Part print with two shaded views. Sizes in mm from the minimum x, y, z corner. Give positions to 0.01 mm unless a question says otherwise; leave off trailing zeros. Loops run counter-clockwise (first coordinate to the right, second up) from the corner with the lowest first, then second, coordinate; pieces in that order, holes last. Notation, with made-up numbers: M 52,7.25 L 76,7.25 A24 ccw 76,38.25 Z; hole C 67,-32.75 d2. An arc over 180 degrees is marked long. Answer as a JSON object with one key per item and string values. Group by question number.
1. Slice it at B-B (x = 56). List the corners of the cut face in (y, z).
2. Drop flat-ended pins along their axis: pin 1 Ø0.8 at (x, y) = (113, 1.5) entering from -Z; pin 2 Ø1 at (y, z) = (1, 44.5) entering from +X; pin 3 Ø1.3 at (y, z) = (1.5, 24) entering from -X. Give the stop position or say it passes through.
3. Drill centre lines: line 1 along X through (y, z) = (1.5, 2.5); line 2 along Z through (x, y) = (106.5, 2.35); line 3 along X through (y, z) = (0.8, 6). Where is each one in solid material? Low to high. Write a range as [from, to].
4. Slice it at A-A (z = 25). List the corners of the cut face in (x, y).
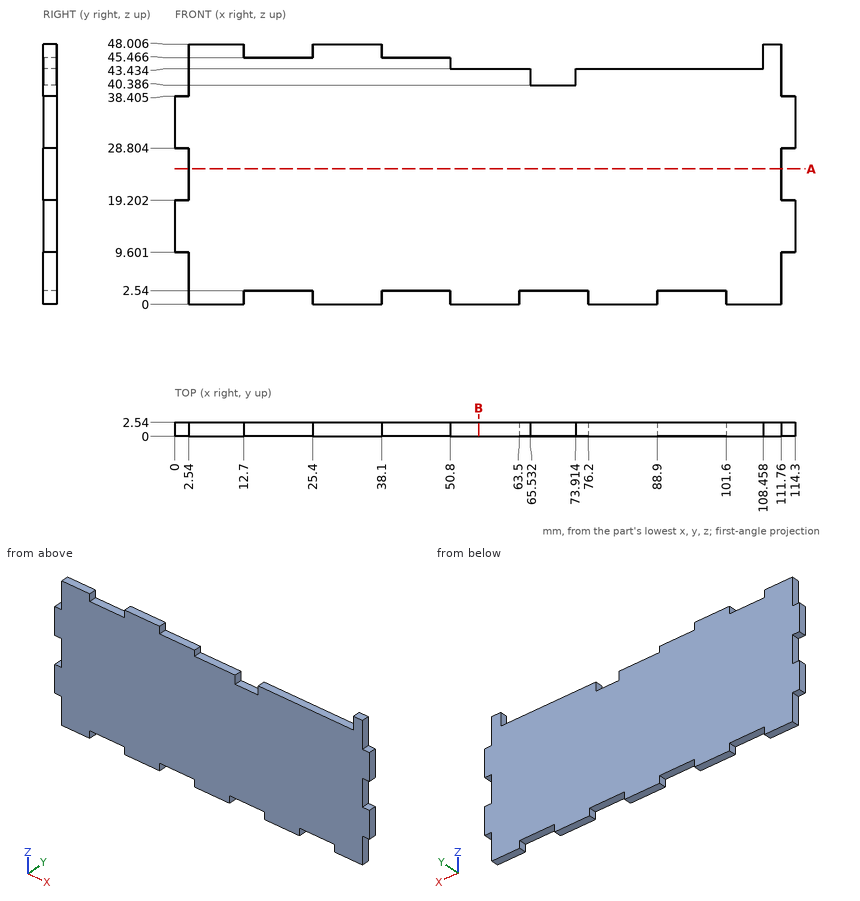
Established:
{
 "1": {"outline": "M 0,0 L 2.54,0 L 2.54,43.43 L 0,43.43 Z"},
 "2": {"pin 1": "stops at z = 9.6", "pin 2": "stops at x = 111.76", "pin 3": "stops at x = 2.54"},
 "3": {"line 1": "x = [2.54, 12.7], [25.4, 38.1], [50.8, 63.5], [76.2, 88.9], [101.6, 111.76]", "line 2": "z = [0, 43.43]", "line 3": "x = [2.54, 111.76]"},
 "4": {"outline": "M 2.54,0 L 111.76,0 L 111.76,2.54 L 2.54,2.54 Z"}
}
